from build123d import *

# Parameters (mm, degrees)
SKETCH1_R      = 3.2999934
EXTRUDE1_DEPTH = 15.875
FILLET1_R      = 7.9375


with BuildPart() as part:
    # Sketch1 → Extrude1 (new body)
    with BuildSketch(Plane.XY):
        Polygon((131.1183814, 88.3896378), (98.8183698, 88.3592086), (98.8183698, 174.2591892), (131.1183814, 174.2591892), align=None)
        with Locations((107.2183784, 102.7091926)):
            Circle(SKETCH1_R, mode=Mode.SUBTRACT)
        with Locations((107.2183784, 159.9092052)):
            Circle(SKETCH1_R, mode=Mode.SUBTRACT)
    extrude(amount=-EXTRUDE1_DEPTH)

    # Fillet1
    fillet1_edges = [part.edges().sort_by_distance(p)[0] for p in [
        (114.9683756, 88.3744232, -15.875),
        (114.9683756, 88.3744232, 0),
        (114.9683756, 174.2591892, -15.875),
        (114.9683756, 174.2591892, 0),
    ]]
    fillet(fillet1_edges, radius=FILLET1_R - 0.0001)  # a hair under: the kernel refuses the full size


solid = part.part
CAD build for the part. Positions are in the model's coordinates, mm. Coordinates: 2 decimals unless noted, no trailing zeros. Loops run counter-clockwise (first coordinate to the right, second up) from the corner with the lowest first, then second, coordinate; pieces in that order, holes last. Notation, with made-up numbers: (59.25, -15.5) - (97.25, -15.5) arc R34 cw to (97.25, 21.5) - close; hole circle Ø2 at (40.25, -30). An arc over 180 degrees is marked (long way). Use one line per item in the form item = value. Start each with the question number.
1) Band-saw the part on C-C (x = 106). State how many separate pieces and enclosed holes the cut face has, and give its area (3 significant figures).
2) Drill centre lines: L1, parallel to Y at x = 104.5, z = -13.5; L2, parallel to X at y = 161.5, z = -11.25; L3, parallel to Y at x = 119, z = -13.25. Where is each one in solid material? Low to high. Write a range as from..to.
3) Band-saw the part on D-D (z = -5). Give the cut face in (x, y).
4) Band-saw the part on B-B (z = -14). Give the cut face in (x, y).
5) Band-saw the part on A-A (y = 158). Give the cut face in (x, z) (3 decimals), and give its area (3 significant figures).
6) Flat gauge pins, fed straight in: pin 1 (4 mm diameter, centred on x = 107.22, y = 159.91, fed in from -Z); pin 2 (1 mm diameter, centred on x = 121.5, z = -1.5, fed in from -Y); pin 3 (3 mm diameter, centred on x = 123.5, z = -11.5, fed in from +Y). Where does each tip first touch, or does it go through?
7) Two-plate mould, pull along Y, no slides. Class faces 1 (the face through (108.74, 99.78, -7.83)), 2 (the face through (98.818, 131, -8)), 3 (the face through (115.19, 172, -2.39)): +Y half, -Y half, draft (parallel to the pull), parting line (faces both ways), or undercut.
Check values:
q1.separate_pieces = 3
q1.enclosed_holes = 0
q1.area = 1,110 mm2
q2.L1 = 90.64..100.84, 104.58..158.04, 161.78..171.98
q2.L2 = 98.82..104.33, 110.11..131.12
q2.L3 = 90.42..172.22
q3.outline = (98.82, 88.92) - (131.12, 88.95) - (131.12, 173.7) - (98.82, 173.7) - close; hole circle Ø6.6 at (107.22, 102.71); hole circle Ø6.6 at (107.22, 159.91)
q4.outline = (98.82, 91.17) - (131.12, 91.2) - (131.12, 171.45) - (98.82, 171.45) - close; hole circle Ø6.6 at (107.22, 102.71); hole circle Ø6.6 at (107.22, 159.91)
q5.outline = (98.818, -15.875) - (104.527, -15.875) - (104.527, 0) - (98.818, 0) - close; (109.91, -15.875) - (131.118, -15.875) - (131.118, 0) - (109.91, 0) - close
q5.area = 427 mm2
q6.pin_1 = through
q6.pin_2 = 91.05
q6.pin_3 = 173.99
q7.face_1 = undercut
q7.face_2 = draft
q7.face_3 = +Y half
